Here's how the part is built. I have some questions about the finished solid (model axes, mm). Face numbers are marked on the shaded views. A direction names the side the tool comes from. Give positions to 0.01 mm unless a question says otherwise; leave off trailing zeros. Order: outer loops, then holes, each group sorted by start corner. A loop starts at its lowest first (then second) coordinate and runs counter-clockwise, first axis right, second up. Notation, with made-up numbers: M 21.25,74 L 51.25,74 A9 cw 51.25,84 Z; hole C -40,67 d2. An arc over 180 degrees is marked long. Use one line per item in the form item = value.
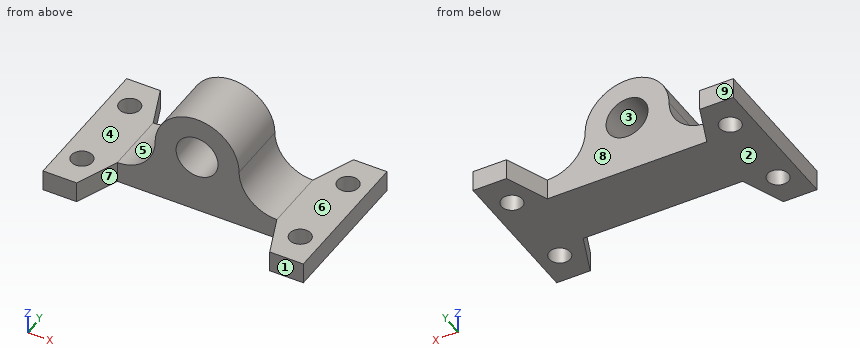
from build123d import *

# Parameters (mm, degrees)
F0_R     = 20
F1_DEPTH = 60
F2_W     = 40
F2_H     = 20
F2_W_2   = 60
F3_DEPTH = 48
F5_DEPTH = 20.001
F7_R     = 10
F8_DEPTH = 20.001


with BuildPart() as f1:
    # F0 (on Front) → F1 (new body)
    with BuildSketch(Plane.XZ):
        with BuildLine():
            ThreePointArc((76, -36), (50.544156, -25.455844), (40, 0))
            ThreePointArc((40, 0), (0, 40), (-40, 0))
            ThreePointArc((-40, 0), (-50.544156, -25.455844), (-76, -36))
            Line((-76, -36), (-76, -56))
            Line((-76, -56), (76, -56))
            Line((76, -56), (76, -36))
        make_face()
        Circle(F0_R, mode=Mode.SUBTRACT)
    extrude(amount=F1_DEPTH)

    # F2 (on face) → F3 (join)
    with BuildSketch(Plane.YZ.offset(76)):
        with Locations((-80, -46)):
            Rectangle(F2_W, F2_H)
        with Locations((20, -46)):
            Rectangle(F2_W, F2_H)
        with Locations((-30, -46)):
            Rectangle(F2_W_2, F2_H)
    extrude(amount=F3_DEPTH)

    # F4 (on face) → F5 (cut, through all)
    with BuildSketch(Plane.XY.offset(-36)):
        Polygon((76, 0), (92, 40), (76, 40), align=None)
        Polygon((76, -100), (92, -100), (76, -60), align=None)
    extrude(amount=-F5_DEPTH, mode=Mode.SUBTRACT)

    # F6: F1 across plane


with BuildPart() as f1_1:
    add(f1.part)
    add(f1.part.mirror(Plane.YZ))

    # F7 (on face) → F8 (cut, through all)
    with BuildSketch(Plane.XY.offset(-36)):
        with Locations((-104, -70)):
            Circle(F7_R)
        with Locations((-104, 10)):
            Circle(F7_R)
    extrude(amount=-F8_DEPTH, mode=Mode.SUBTRACT)

    # F9: F1 across plane


with BuildPart() as f1_2:
    add(f1_1.part)
    add(f1_1.part.mirror(Plane.YZ), mode=Mode.INTERSECT)


solid = f1_2.part
Q1. On a 3-axis mill with a long thin cutter (end or side, diameter ignored), from which of +Z, -Z, +X, -X, +Y, -Y can I reach the whole of each face in a straight line? I mean the marked faces 5, 6, 7, 8 and 9. Say none if no direction works.
Found:
face_5 = +Z, -X, +Y, -Y
face_6 = +Z, +X, +Y, -Y
face_7 = +Z, -Z, -Y
face_8 = +Z, -Z, +Y
face_9 = +Z, -Z, +X, -X, +Y
Q2. I want a section at B-B on y = 10. Write out the boundary of the cut face in (x, z).
Found:
outline = M -124,-56 L -114,-56 L -114,-36 L -124,-36 Z; M -94,-56 L -80,-56 L -80,-36 L -94,-36 Z; M 80,-56 L 94,-56 L 94,-36 L 80,-36 Z; M 114,-56 L 124,-56 L 124,-36 L 114,-36 Z
Q3. I want a section at A-A on x = 104. Write out the boundary of the cut face in (y, z).
Found:
outline = M -100,-56 L -80,-56 L -80,-36 L -100,-36 Z; M -60,-56 L 0,-56 L 0,-36 L -60,-36 Z; M 20,-56 L 40,-56 L 40,-36 L 20,-36 Z
Q4. I'm going to push flat-ended pins straight in: pin 1 Ø4 at (y, z) = (-40, 20.5) entering from +X; pin 2 Ø24 at (x, y) = (-89, -2.5) entering from +Z. Where does each tip first touch, or does it pass through?
Found:
pin_1 = 35.46
pin_2 = -36
Q5. Thinking about a two-plate mould opening in Z: for the marked faces 1, 2, 3 and 4, which applies, +Z half, -Z half, draft (parallel to the pull), parting line (faces both ways), or undercut?
Found:
face_1 = draft
face_2 = -Z half
face_3 = undercut
face_4 = +Z half
Q6. I want a section at C-C on y = -6. Write out the boundary of the cut face in (x, z), then the cut area to 3 significant figures.
Found:
outline = M -124,-56 L 124,-56 L 124,-36 L 76,-36 A36 cw 40,0 A40 ccw -40,0 A36 cw -76,-36 L -124,-36 Z; hole C 0,0 d40
area = 9,650 mm²
Q7. I need wall thicknesses on L1, parallel to Y at x = 104, z = -45.5; L2, parallel to X at y = 6, z = -44; L3, parallel to Y at x = 60, z = -35. Which ranges of each line are inside material? Lowest first, please.
Found:
L1 = -100 to -80, -60 to 0, 20 to 40
L2 = -124 to -113.17, -94.83 to -78.4, 78.4 to 94.83, 113.17 to 124
L3 = -60 to 0
Q8. I want a section at D-D on z = -9.5. Write out the boundary of the cut face in (x, y).
Found:
outline = M -41.28,-60 L -17.6,-60 L -17.6,0 L -41.28,0 Z; M 17.6,-60 L 41.28,-60 L 41.28,0 L 17.6,0 Z
